Input: part model. Units: mm. Frame: model coordinates. Give positions to 0.01 mm unless a question says otherwise; leave off trailing zeros. Write each loop counter-clockwise with the first axis right and the second up, starting at its lowest first coordinate (ties: lowest second). Pieces come first, ordered by that corner, then holes.
```python
from build123d import *

# Parameters (mm, degrees)
F0_R     = 3.5
F1_DEPTH = 3


# Not quite as in the source:
# - a feature names something its author has since deleted; it is built from what else it names


with BuildPart() as f1:
    # F0 (on Top) → F1 (new body)
    with BuildSketch(Plane.XY):
        with BuildLine():
            Line((-103.8872403759, 50.9688953831), (-101.9313409925, 50.9688953831))
            Line((-101.9313409925, 50.9688953831), (-99.975441609, 50.9688953831))
            ThreePointArc((-99.975441609, 50.9688953831), (-101.9313409925, 51.0198679723), (-103.8872403759, 50.9688953831))
        make_face()
        with BuildLine():
            ThreePointArc((-105.128088395, 44.1726214205), (-103.7275117352, 47.6637957311), (-101.9313409925, 50.9688953831))
            Line((-101.9313409925, 50.9688953831), (-103.8872403759, 50.9688953831))
            ThreePointArc((-103.8872403759, 50.9688953831), (-118.4470490216, 47.1928769199), (-130.3569155648, 38.005852257))
            ThreePointArc((-130.3569155648, 38.005852257), (-128.876069776, 34.6235055457), (-127.0483694881, 31.4152840472))
            ThreePointArc((-127.0483694881, 31.4152840472), (-131.6855143995, 21.6924682926), (-132.6995872702, 10.9682939496))
            ThreePointArc((-132.6995872702, 10.9682939496), (-136.152020588, 12.3518590173), (-139.4313409925, 14.1067395817))
            Line((-139.4313409925, 14.1067395817), (-139.4313409925, 11.5129959997))
            ThreePointArc((-139.4313409925, 11.5129959997), (-135.8835245013, -2.5724504886), (-127.2555101816, -14.2576622337))
            ThreePointArc((-127.2555101816, -14.2576622337), (-123.8698155437, -12.8388675837), (-120.6478658456, -11.079621557))
            ThreePointArc((-120.6478658456, -11.079621557), (-109.6296820224, -16.4254775309), (-97.3998915176, -17.0663948921))
            ThreePointArc((-97.3998915176, -17.0663948921), (-98.4971319541, -20.6192094649), (-99.975441609, -24.0311046169))
            ThreePointArc((-99.975441609, -24.0311046169), (-85.5790985856, -20.3346504467), (-73.7446837693, -11.342148468))
            ThreePointArc((-73.7446837693, -11.342148468), (-75.1429207557, -7.8890051383), (-76.9083449574, -4.6083736574))
            ThreePointArc((-76.9083449574, -4.6083736574), (-71.9248057865, 6.2200450283), (-71.4154696243, 18.1293225284))
            ThreePointArc((-71.4154696243, 18.1293225284), (-67.8499010769, 16.9668747828), (-64.4313409925, 15.4247947665))
            ThreePointArc((-64.4313409925, 15.4247947665), (-67.9189218222, 29.3821252434), (-76.3988312093, 41.0037185452))
            ThreePointArc((-76.3988312093, 41.0037185452), (-79.9768515125, 39.773669955), (-83.3966724505, 38.1550058214))
            ThreePointArc((-83.3966724505, 38.1550058214), (-93.6932659385, 43.219056827), (-105.128088395, 44.1726214205))
        make_face()
        with BuildLine():
            ThreePointArc((-116.8786483854, -8.4112257418), (-114.7452282061, -6.5377141597), (-112.7675725108, -4.500459816))
            ThreePointArc((-112.7675725108, -4.500459816), (-104.8400955118, -7.312365092), (-96.445234408, -6.785098651))
            ThreePointArc((-96.445234408, -6.785098651), (-96.3945126034, -9.6374635235), (-96.5828731928, -12.4840541783))
            ThreePointArc((-96.5828731928, -12.4840541783), (-107.144920689, -12.5114873217), (-116.8786483854, -8.4112257418))
        make_face(mode=Mode.SUBTRACT)
        with BuildLine():
            ThreePointArc((-97.1633932868, -1.5770140117), (-103.489663028, -2.237292801), (-109.5628503108, -0.3467761664))
            ThreePointArc((-109.5628503108, -0.3467761664), (-108.1146014235, 2.0457215346), (-106.8582364184, 4.544324557))
            ThreePointArc((-106.8582364184, 4.544324557), (-102.9079011749, 3.321551239), (-98.7968737544, 3.768515076))
            ThreePointArc((-98.7968737544, 3.768515076), (-97.870198127, 1.1293444599), (-97.1633932868, -1.5770140117))
        make_face(mode=Mode.SUBTRACT)
        with BuildLine():
            ThreePointArc((-87.020290304, 18.643185886), (-86.1794714129, 12.4732450474), (-87.7904785909, 6.4582801904))
            ThreePointArc((-87.7904785909, 6.4582801904), (-90.2129680661, 7.8584356684), (-92.7417733998, 9.0559473403))
            ThreePointArc((-92.7417733998, 9.0559473403), (-91.7456646982, 13.0514491022), (-92.4114813686, 17.1150626462))
            ThreePointArc((-92.4114813686, 17.1150626462), (-89.7469190596, 17.9886089148), (-87.020290304, 18.643185886))
        make_face(mode=Mode.SUBTRACT)
        with BuildLine():
            ThreePointArc((-79.6045613776, -0.8026360965), (-81.5030217359, 1.3342277264), (-83.5732367524, 3.3051535278))
            ThreePointArc((-83.5732367524, 3.3051535278), (-81.0808826805, 11.1066871006), (-81.7647527708, 19.2680642275))
            ThreePointArc((-81.7647527708, 19.2680642275), (-78.8888619154, 19.2681720991), (-76.0229262651, 19.0290882807))
            ThreePointArc((-76.0229262651, 19.0290882807), (-75.8548608571, 8.7594492912), (-79.6045613776, -0.8026360965))
        make_face(mode=Mode.SUBTRACT)
        with BuildLine():
            ThreePointArc((-124.2925325258, 27.6864483354), (-122.366283457, 25.5897237243), (-120.2765526126, 23.655889562))
            ThreePointArc((-120.2765526126, 23.655889562), (-122.6767843834, 16.6229750116), (-122.4752234892, 9.1944911263))
            ThreePointArc((-122.4752234892, 9.1944911263), (-125.3358583127, 9.3662040749), (-128.1716299117, 9.7798662184))
            ThreePointArc((-128.1716299117, 9.7798662184), (-127.8289740179, 19.0790916737), (-124.2925325258, 27.6864483354))
        make_face(mode=Mode.SUBTRACT)
        with BuildLine():
            ThreePointArc((-116.0346336158, 20.5547864365), (-113.602585651, 19.1733015065), (-111.068333377, 17.9896954377))
            ThreePointArc((-111.068333377, 17.9896954377), (-112.0801205218, 14.4304238708), (-111.7547699117, 10.7444675099))
            ThreePointArc((-111.7547699117, 10.7444675099), (-114.4574555109, 10.0161737122), (-117.2111759917, 9.514232662))
            ThreePointArc((-117.2111759917, 9.514232662), (-117.6257828154, 15.1413817681), (-116.0346336158, 20.5547864365))
        make_face(mode=Mode.SUBTRACT)
        with Locations((-101.9313409925, 13.4688953831)):
            Circle(F0_R, mode=Mode.SUBTRACT)
        with BuildLine():
            ThreePointArc((-106.3733358176, 28.6142377963), (-100.6487081208, 29.1999973076), (-95.0945804167, 27.6946262842))
            ThreePointArc((-95.0945804167, 27.6946262842), (-96.6062830352, 25.3254140346), (-97.9178620412, 22.8398211472))
            ThreePointArc((-97.9178620412, 22.8398211472), (-101.4213565394, 23.6503578923), (-104.988310348, 23.1939764279))
            ThreePointArc((-104.988310348, 23.1939764279), (-105.7981495503, 25.8741269811), (-106.3733358176, 28.6142377963))
        make_face(mode=Mode.SUBTRACT)
        with BuildLine():
            ThreePointArc((-87.3838790757, 35.6168761154), (-89.634828263, 33.8018778137), (-91.7240079261, 31.8027981717))
            ThreePointArc((-91.7240079261, 31.8027981717), (-99.0699795968, 34.2567343942), (-106.8057550879, 33.8787392584))
            ThreePointArc((-106.8057550879, 33.8787392584), (-106.6786212529, 36.7532837824), (-106.296701705, 39.6051790629))
            ThreePointArc((-106.296701705, 39.6051790629), (-96.4636690625, 39.3969933158), (-87.3838790757, 35.6168761154))
        make_face(mode=Mode.SUBTRACT)
        with BuildLine():
            Line((-139.4313409925, 14.1067395817), (-139.4313409925, 15.4247947665))
            ThreePointArc((-139.4313409925, 15.4247947665), (-139.4594284478, 14.7796945074), (-139.4764192758, 14.1342066599))
            ThreePointArc((-139.4764192758, 14.1342066599), (-139.4538855016, 14.1204643119), (-139.4313409925, 14.1067395817))
        make_face()
        with BuildLine():
            Line((-139.4313409925, 11.5129959997), (-139.4313409925, 14.1067395817))
            ThreePointArc((-139.4313409925, 14.1067395817), (-139.4538855016, 14.1204643119), (-139.4764192758, 14.1342066599))
            ThreePointArc((-139.4764192758, 14.1342066599), (-139.4767618846, 12.8232078208), (-139.4313409925, 11.5129959997))
        make_face()
    extrude(amount=F1_DEPTH)


solid = f1.part
```
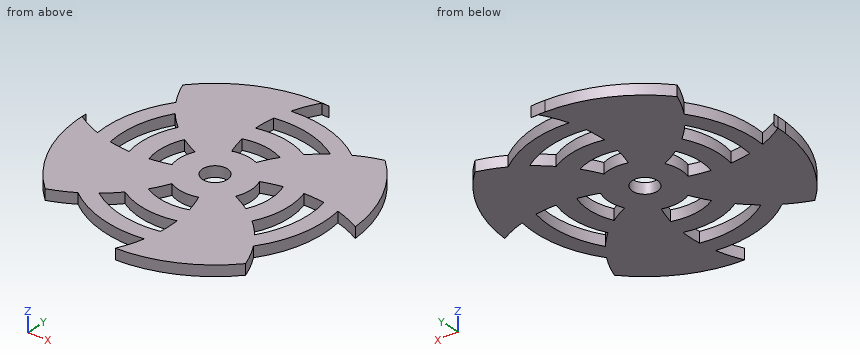
Item 1: Section A-A (x = -125.5). Return loops of the section in (y, z), and give its area (3 significant figures).
Item 2: Section B-B (z = 2.05). Give the number of separate pieces and of enclosed holes in the cut face, and give its area (3 significant figures).
Item 3: Pin query (flat end, axial travel): pin 1 (1.1 mm diameter, centred on y = 14.5, z = 2, fed in from +X); pin 2 (1 mm diameter, centred on x = -112.5, y = -11, fed in from -Z); pin 3 (4 mm diameter, centred on x = -101.93, y = 13.47, fed in from +Z). Return the tip coordinate at first contact, or that it passes through.
Item 4: Ray query, line 1 (Y direction, x = -113, z = 1.1); line 2 (X direction, y = 25, z = 0.3); line 3 (X direction, y = 27.5, z = 0.45). Return the intervals inside material, ascending.
Item 5: Section C-C (y = -15.5). Return loops of the section in (x, z).
Solved:
1. outline: (-13.57, 0) - (9.38, 0) - (9.38, 3) - (-13.57, 3) - close; (25.58, 0) - (42.7, 0) - (42.7, 3) - (25.58, 3) - close
1. area: 120 mm2
2. separate pieces: 1
2. enclosed holes: 9
2. area: 3,080 mm2
3. pin 1: stops at x = -71.07
3. pin 2: stops at z = 0
3. pin 3: passes through
4. line 1: y = -15.35 to -10.61, -4.76 to 10.38, 18.87 to 49.35
4. line 2: x = -130.57 to -125.79, -121.76 to -105.56, -96.79 to -66.19
4. line 3: x = -129.43 to -124.41, -124.13 to -106.17, -95.23 to -67.1
5. outline: (-112.6, 0) - (-78.04, 0) - (-78.04, 3) - (-112.6, 3) - close
